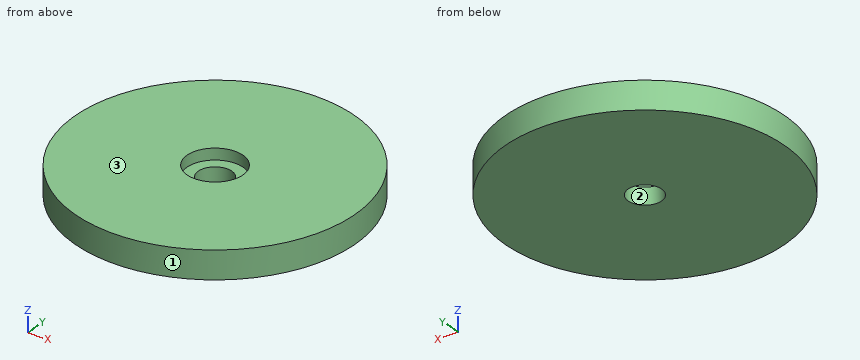
Autodesk Fusion 360 part; units mm, degrees
sketch "Sketch1" plane through (0, 0, 0) normal (0, 0, 1) x (1, 0, 0)
  circle A0 centre (0, 0) radius 25
  dimension "d1" = 50
extrude "Extrude1" add sketch "Sketch1" along normal blind 5
sketch "Sketch2" plane through (0, 0, 5) normal (0, 0, 1) x (-1, 0, 0)
  circle A0 centre (0, 0) radius 25
  circle A1 centre (0, 0) radius 5
  dimension "d4" = 10
extrude "Extrude3" cut sketch "Sketch2" against normal blind 2 contours A1
sketch "Sketch3" plane through (0, 0, 5) normal (0, 0, 1) x (-1, 0, 0)
  circle A0 centre (0, 0) radius 3
  dimension "d9" = 6
extrude "Extrude4" cut sketch "Sketch3" against normal blind 5
The listing builds one solid part. Answer for the finished solid, in the listing's coordinates (mm). Face numbers are marked on the shaded views. Coordinates: 2 decimals unless noted, no trailing zeros. Loops run counter-clockwise (first coordinate to the right, second up) from the corner with the lowest first, then second, coordinate; pieces in that order, holes last. Notation, with made-up numbers: (18, 10.5) - (34, 10.5) arc R21 ccw to (34, 24.5) - close; hole circle Ø4 at (-35, -11.75). An arc over 180 degrees is marked (long way). Use a Markdown table: item, result. Add a question column.
1) The part is cut by section A-A, the plane x = 0. Give the vertices of the cut face in (y, z).
2) The mould has two halves that part along Y. Classify the marked faces 1, 2 and 3: released by +Y, released by -Y, zero draft, split by the parting line, or undercut.
3) The part is cut by section C-C, the plane z = 4.35. Give the vertices of the cut face in (x, y), and give its area (3 significant figures).
4) Given pin 1 (1.5 mm diameter, centred on x = 7, z = 4, fed in from +Y); pin 2 (13 mm diameter, centred on x = 0, y = 0, fed in from -Z); pin 3 (1 mm diameter, centred on x = 1.5, z = 2.5, fed in from -Y); pin 4 (2 mm diameter, centred on y = -15, z = 1, fed in from -X), each flat-ended and moving along its own axis, determine where each tip first touches the part or whether it passes through.
5) The part is cut by section D-D, the plane x = -15. Give the vertices of the cut face in (y, z).
6) Find the intervals of material crossed by line 1 (Y direction, x = 0, z = 2.4); line 2 (Y direction, x = 0, z = 4.3); line 3 (X direction, y = -2.5, z = 2.75), in increasing order.
Here are the results:
| question | item | result |
|---|---|---|
| 1 | outline | (-25, 0) - (-3, 0) - (-3, 3) - (-5, 3) - (-5, 5) - (-25, 5) - close; (3, 0) - (25, 0) - (25, 5) - (5, 5) - (5, 3) - (3, 3) - close |
| 2 | face 1 | split by the parting line |
| 2 | face 2 | undercut |
| 2 | face 3 | zero draft |
| 3 | outline | circle Ø50 at (0, 0); hole circle Ø10 at (0, 0) |
| 3 | area | 1,880 mm^2 |
| 4 | pin 1 | stops at y = 24.21 |
| 4 | pin 2 | stops at z = 0 |
| 4 | pin 3 | stops at y = -24.98 |
| 4 | pin 4 | stops at x = -20.71 |
| 5 | outline | (-20, 0) - (20, 0) - (20, 5) - (-20, 5) - close |
| 6 | line 1 | y = -25 to -3, 3 to 25 |
| 6 | line 2 | y = -25 to -5, 5 to 25 |
| 6 | line 3 | x = -24.87 to -1.66, 1.66 to 24.87 |
